```python
from build123d import *

# Parameters (mm, degrees)
F0_W     = 70
F0_H     = 100
F1_DEPTH = 9.5
F2_W     = 43.5
F2_H     = 7
F3_DEPTH = 10
F4_W     = 26.9
F4_H     = 4.6
F4_W_2   = 13
F5_DEPTH = 10


with BuildPart() as f1:
    # F0 (on Top) → F1 (new body)
    with BuildSketch(Plane.XY):
        Rectangle(F0_W, F0_H)
    extrude(amount=F1_DEPTH)

    # F2 (on face) → F3 (cut)
    with BuildSketch(Plane(origin=(0, 50, 0), x_dir=(-1, 0, 0), z_dir=(0, 1, 0))):
        with Locations((-4.75, 3.5)):
            Rectangle(F2_W, F2_H)
    extrude(amount=-F3_DEPTH, mode=Mode.SUBTRACT)

    # F4 (on face) → F5 (join)
    with BuildSketch(Plane(origin=(0, 40, 0), x_dir=(-1, 0, 0), z_dir=(0, 1, 0))):
        with Locations((-11.85, 3.5)):
            Rectangle(F4_W, F4_H)
        with Locations((9.3, 3.5)):
            Rectangle(F4_W_2, F4_H)
    extrude(amount=F5_DEPTH)


solid = f1.part
```
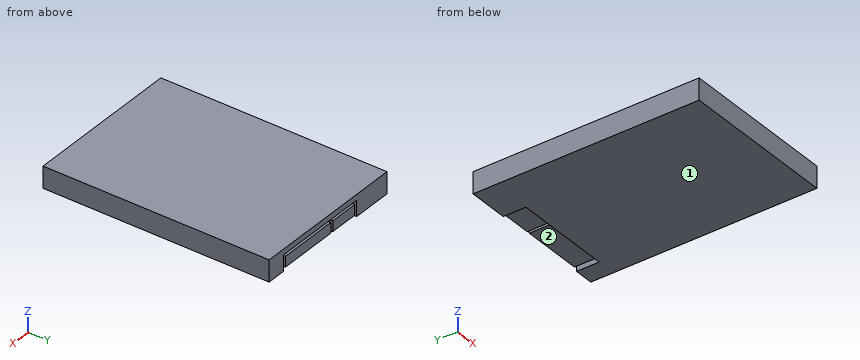
Verification items for the finished model (mm, model axes). Face numbers are marked on the shaded views. A direction names the side the tool comes from. Round coordinates to 2 decimals unless told otherwise and drop trailing zeros. Write each loop counter-clockwise with the first axis right and the second up, starting at its lowest first coordinate (ties: lowest second). Pieces come first, ordered by that corner, then holes.
1. Access from +Z, -Z, +X, -X, +Y, -Y to the whole of each face (thin tool, end or side, straight path). Record for the marked faces 1 and 2.
2. Scan lines: L1, parallel to X at y = 44, z = 2.5; L2, parallel to Y at x = 15, z = 6.75. Record each from-to range of solid material in increasing order.
3. Section check A-A on x = -0.5. Enter the section's corners in (y, z).
4. Gauge pin test, flat end, axial feed: P1, Ø3, axis at x = -5.5, y = 46, coming from the -Z side. Record the tip position at first contact, or that the pin passes through.
Answer:
1. face 1: -Z, +X, -X, +Y, -Y
1. face 2: -Z, +Y
2. L1: x = -35 to -17, -15.8 to -2.8, -1.6 to 25.3, 26.5 to 35
2. L2: y = -50 to 40
3. outline: (-50, 0) - (40, 0) - (40, 1.2) - (50, 1.2) - (50, 5.8) - (40, 5.8) - (40, 7) - (50, 7) - (50, 9.5) - (-50, 9.5) - close
4. P1: stops at z = 1.2
